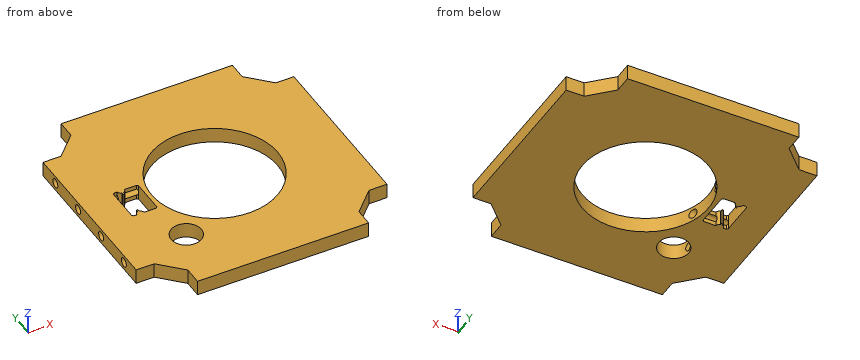
Autodesk Inventor part; units mm, degrees
ref_plane "Work Plane1" through (0, 0, 10) normal (0, 0, 1) x (1, 0, 0)
ref_plane "YZ Plane" through (0, 0, 0) normal (1, 0, 0) x (0, 1, 0)
ref_plane "XZ Plane" through (0, 0, 0) normal (0, 1, 0) x (-1, 0, 0)
ref_plane "Work Plane1" through (0, 0, 10) normal (0, 0, 1) x (1, 0, 0)
sketch "Sketch1" plane through (0, 0, 10) normal (0, 0, 1) x (1, 0, 0)
  line L0 (-4.0299, -0.3538) -> (-2.2322, 1.4439) construction
  arc A0 (-1.4439, 2.2322) -> (-2.2322, 1.4439) centre (-0.9299, 0.9299) ccw construction
  line L1 (-1.4439, 2.2322) -> (0.3538, 4.0299) construction
  line L2 (-37.8299, 42.8299) -> (-37.8299, 37.8299) construction
  line L3 (-37.8299, 37.8299) -> (-42.9208, 37.8299) construction
  line L4 (-37.8299, 42.2137) -> (-37.8299, 45.8299) construction
  line L5 (-37.8299, 45.8299) -> (-4.0299, 45.8299) construction
  line L6 (-4.0299, 45.8299) -> (-4.0299, 42.2137) construction
  line L7 (-4.0299, 4.0299) -> (0.3538, 4.0299)
  circle A1 centre (-20.9299, 20.9299) radius 17.5
  line L8 (-20.9299, 58.9723) -> (17.1124, 20.9299) construction
  line L9 (17.1124, 20.9299) -> (-20.9299, -17.1124) construction
  line L10 (-20.9299, -17.1124) -> (-58.9723, 20.9299) construction
  line L11 (-58.9723, 20.9299) -> (-20.9299, 58.9723) construction
  line L12 (-20.9299, 58.9723) -> (-20.9299, -17.1124) construction
  line L13 (17.1124, 20.9299) -> (-58.9723, 20.9299) construction
  line L14 (-20.9299, 58.9723) -> (32.8701, 58.9723) construction
  line L15 (-43.4299, 43.4299) -> (1.5701, 43.4299) construction
  line L16 (1.5701, 43.4299) -> (1.5701, -1.5701) construction
  line L17 (1.5701, -1.5701) -> (-43.4299, -1.5701) construction
  line L18 (-43.4299, -1.5701) -> (-43.4299, 43.4299) construction
  line L19 (-43.4299, 43.4299) -> (1.5701, -1.5701) construction
  line L20 (1.5701, 43.4299) -> (-43.4299, -1.5701) construction
  line L21 (-43.4299, 5.3876) -> (-43.4299, 36.4723)
  line L22 (-43.4299, 36.4723) -> (-36.4723, 43.4299)
  line L23 (-36.4723, 43.4299) -> (-5.3876, 43.4299)
  line L24 (-5.3876, 43.4299) -> (1.5701, 36.4723)
  line L25 (1.5701, 36.4723) -> (1.5701, 5.3876)
  line L26 (1.5701, 5.3876) -> (-5.3876, -1.5701)
  line L27 (-5.3876, -1.5701) -> (-36.4723, -1.5701)
  line L28 (-36.4723, -1.5701) -> (-43.4299, 5.3876)
  line L29 (-4.0299, 42.2137) -> (-37.8299, 42.2137)
  line L30 (-4.0299, -0.3538) -> (-4.0299, 4.0299)
  circle A2 centre (-20.9299, 20.9299) radius 1.5
  line L31 (-10.9299, 10.9299) -> (-30.9299, 10.9299) construction
  line L32 (-30.9299, 10.9299) -> (-30.9299, 30.9299) construction
  line L33 (-30.9299, 30.9299) -> (-10.9299, 30.9299) construction
  line L34 (-10.9299, 30.9299) -> (-10.9299, 10.9299) construction
  line L35 (-10.9299, 10.9299) -> (-30.9299, 30.9299) construction
  line L36 (-30.9299, 10.9299) -> (-10.9299, 30.9299) construction
  circle A3 centre (-30.9299, 30.9299) radius 1.4
  circle A4 centre (-30.9299, 10.9299) radius 1.4
  circle A5 centre (-10.9299, 10.9299) radius 1.4
  line L37 (-45.8299, 37.8299) -> (-42.0723, 37.8299) construction
  line L38 (-42.1723, 37.7299) -> (-45.8299, 37.7299)
  line L39 (-45.8299, 37.7299) -> (-45.8299, 4.1299)
  line L40 (-45.8299, 4.1299) -> (-42.1723, 4.1299)
  line L41 (-42.1723, 4.1299) -> (-42.1723, 37.7299)
  line L42 (-45.8299, 4.0299) -> (-42.0723, 4.0299) construction
  line L43 (-45.8299, 37.8299) -> (-42.0723, 37.8299)
  line L44 (-37.7299, 45.8299) -> (-4.1299, 45.8299)
  line L45 (-4.1299, 45.8299) -> (-4.1299, 42.1723)
  line L46 (-4.1299, 42.1723) -> (-37.7299, 42.1723)
  line L47 (-37.7299, 42.1723) -> (-37.7299, 45.8299)
  line L48 (0.4701, 37.8299) -> (0.4701, 4.0299) construction
  line L49 (0.4701, 4.0299) -> (3.9701, 4.0299) construction
  line L50 (3.9701, 37.8299) -> (3.9701, 4.0299) construction
  line L51 (0.4701, 37.8299) -> (3.9701, 37.8299) construction
  line L52 (-45.8299, -3.9701) -> (-4.0299, -3.9701) construction
  line L53 (0.3124, 37.7299) -> (3.9701, 37.7299)
  line L54 (3.9701, 37.7299) -> (3.9701, 4.1299)
  line L55 (3.9701, 4.1299) -> (0.3124, 4.1299)
  line L56 (0.3124, 4.1299) -> (0.3124, 37.7299)
  line L57 (-4.1713, -0.3538) -> (-37.7299, -0.3538)
  line L58 (-37.7299, -0.3538) -> (-37.7299, -3.9701)
  line L59 (-37.7299, -3.9701) -> (-4.1713, -3.9701)
  line L60 (-4.1713, -3.9701) -> (-4.1713, -0.3538)
  point P0 (-37.8299, 4.0299)
  dimension "d18" = 53.8
  dimension "d19" = 45
  dimension "d20" = 53.8
  dimension "d21" = 45
  dimension "d22" = 45
  dimension "d30" = 20
  dimension "d31" = 20
  dimension "d32" = 2.8
  dimension "d33" = 2.8
  dimension "d34" = 2.8
  dimension "d35" = 3
  dimension "d36" = 0.1
  dimension "d37" = 0.1
  dimension "d38" = 0.1
  dimension "d39" = 0.1
extrude "Extrusion1" add sketch "Sketch1" along normal blind 3 contours L30 L26 L57 L28 L41 L22 L46 L24 L56 L7 | L7 L26 L30 | L56 L24 L25 L26 | L26 L25 L24 L53 L54 L55 | L60 L59 L58 L57 L28 L27 L26 | L26 L27 L28 L57 | L46 L22 L29 L24 | L24 L29 L45 | L40 L39 L38 L22 L21 L28 | L28 L21 L22 L41 | L29 L22 L23 L24 | L24 L23 L22 L29 L47 L44 L45 | L47 L29 L22 | A1 | A2 | A3 | A4 | A5
sketch "Skizze4" plane through (0, 0, 13) normal (0, 0, 1) x (1, 0, 0)
  line L0 (-37.7299, 42.1723) -> (-42.1723, 37.7299)
  line L1 (-42.1723, 37.7299) -> (-45.8299, 37.7299)
  line L2 (-45.8299, 37.7299) -> (-45.8299, 4.1299) construction
  line L3 (-45.8299, 4.1299) -> (-42.1723, 4.1299)
  line L4 (-42.1723, 4.1299) -> (-37.6885, -0.3538)
  line L5 (-37.6885, -0.3538) -> (-37.7299, -0.3538)
  line L6 (-37.7299, -0.3538) -> (-37.7299, -3.9701)
  line L7 (-37.7299, -3.9701) -> (-4.1713, -3.9701) construction
  line L8 (-4.1713, -3.9701) -> (-4.1713, -0.3538)
  line L9 (-4.1713, -0.3538) -> (0.3124, 4.1299)
  line L10 (0.3124, 4.1299) -> (3.9701, 4.1299)
  line L11 (3.9701, 4.1299) -> (3.9701, 37.7299) construction
  line L12 (3.9701, 37.7299) -> (0.3124, 37.7299)
  line L13 (0.3124, 37.7299) -> (-4.1299, 42.1723)
  line L14 (-4.1299, 42.1723) -> (-4.1299, 45.8299)
  line L15 (-4.1299, 45.8299) -> (-37.7299, 45.8299) construction
  line L16 (-37.7299, 45.8299) -> (-37.7299, 42.1723)
  line L17 (-37.9299, 46.0299) -> (-3.9299, 46.0299) construction
  line L18 (-3.9299, 46.0299) -> (-3.9299, 42.2551)
  line L19 (-3.9299, 42.2551) -> (0.3953, 37.9299)
  line L20 (0.3953, 37.9299) -> (4.1701, 37.9299)
  line L21 (4.1701, 37.9299) -> (4.1701, 3.9299) construction
  line L22 (4.1701, 3.9299) -> (0.3953, 3.9299)
  line L23 (0.3953, 3.9299) -> (-3.9713, -0.4367)
  line L24 (-3.9713, -0.4367) -> (-3.9713, -4.1701)
  line L25 (-3.9713, -4.1701) -> (-37.9299, -4.1701) construction
  line L26 (-37.9299, -4.1701) -> (-37.9299, -0.3953)
  line L27 (-37.9299, -0.3953) -> (-42.2551, 3.9299)
  line L28 (-42.2551, 3.9299) -> (-46.0299, 3.9299)
  line L29 (-46.0299, 3.9299) -> (-46.0299, 37.9299) construction
  line L30 (-46.0299, 37.9299) -> (-42.2551, 37.9299)
  line L31 (-42.2551, 37.9299) -> (-37.9299, 42.2551)
  line L32 (-37.9299, 42.2551) -> (-37.9299, 46.0299)
  line L33 (-45.8299, 37.7299) -> (-45.8299, 37.9299)
  line L34 (-4.1299, 45.8299) -> (-37.7299, 45.8299)
  line L35 (-37.7299, 45.8299) -> (-37.9299, 45.8299)
  line L36 (-4.1299, 45.8299) -> (-3.9299, 45.8299)
  line L37 (3.9701, 37.7299) -> (3.9701, 37.9299)
  line L38 (3.9701, 4.1299) -> (3.9701, 37.7299)
  line L39 (3.9701, 4.1299) -> (3.9701, 3.9299)
  line L40 (-4.1713, -3.9701) -> (-3.9713, -3.9701)
  line L41 (-37.7299, -3.9701) -> (-37.9299, -3.9701)
  line L42 (-45.8299, 4.1299) -> (-45.8299, 3.9299)
  point P0 (0, 0)
  dimension "d40" = 0.2
extrude "IM_offset" add sketch "Skizze4" against normal up to surface (3 mm away)
ref_plane "Arbeitsebene5" through (-20.9299, 3.9299, 10) normal (1, 0, 0) x (0, 0, -1)
ref_plane "Arbeitsebene6" through (-37.9299, 20.9299, 10) normal (0, 1, 0) x (1, 0, 0)
sketch "Skizze25" plane through (0, 0, 13) normal (0, 0, 1) x (1, 0, 0)
  arc A0 (-37.9299, 18.0899) -> (-38.4737, 17.4299) centre (-37.6799, 17.3299) ccw
  line L0 (-37.9299, 18.0899) -> (-37.9299, 18.5899)
  line L1 (-37.9299, 18.5899) -> (-37.4299, 18.5899)
  line L2 (-37.4299, 18.5899) -> (-37.4299, 18.0899)
  arc A1 (-36.8862, 17.4299) -> (-37.4299, 18.0899) centre (-37.6799, 17.3299) ccw
  line L3 (-36.8862, 17.4299) -> (-34.5799, 17.4299)
  line L4 (-34.5799, 17.4299) -> (-34.3799, 17.6299)
  line L5 (-34.3799, 17.6299) -> (-34.3799, 24.2299)
  line L6 (-34.3799, 24.2299) -> (-34.5799, 24.4299)
  line L7 (-34.5799, 24.4299) -> (-36.8862, 24.4299)
  arc A2 (-37.4299, 23.77) -> (-36.8862, 24.4299) centre (-37.6799, 24.5299) ccw
  line L8 (-37.4299, 23.77) -> (-37.4299, 23.27)
  line L9 (-37.4299, 23.27) -> (-37.9299, 23.27)
  line L10 (-37.9299, 23.27) -> (-37.9299, 23.77)
  arc A3 (-38.4737, 24.4299) -> (-37.9299, 23.77) centre (-37.6799, 24.5299) ccw
  line L11 (-38.4737, 24.4299) -> (-38.9799, 24.4299)
  line L12 (-38.9799, 24.4299) -> (-39.1799, 24.2299)
  line L13 (-39.1799, 24.2299) -> (-39.1799, 17.6299)
  line L14 (-39.1799, 17.6299) -> (-38.9799, 17.4299)
  line L15 (-38.9799, 17.4299) -> (-38.4737, 17.4299)
  line L16 (-34.2799, 24.2713) -> (-34.2799, 17.5885)
  line L17 (-34.2799, 17.5885) -> (-34.5385, 17.3299)
  line L18 (-34.5385, 17.3299) -> (-36.9799, 17.3299)
  arc A4 (-36.9799, 17.3299) -> (-37.5299, 18.0137) centre (-37.6799, 17.3299) ccw
  line L19 (-37.5299, 18.0137) -> (-37.5299, 18.4899)
  line L20 (-37.5299, 18.4899) -> (-37.8299, 18.4899)
  line L21 (-37.8299, 18.4899) -> (-37.8299, 18.0137)
  arc A5 (-37.8299, 18.0137) -> (-38.3799, 17.3299) centre (-37.6799, 17.3299) ccw
  line L22 (-38.3799, 17.3299) -> (-39.0213, 17.3299)
  line L23 (-39.0213, 17.3299) -> (-39.2799, 17.5885)
  line L24 (-39.2799, 17.5885) -> (-39.2799, 24.2713)
  line L25 (-39.2799, 24.2713) -> (-39.0213, 24.5299)
  line L26 (-39.0213, 24.5299) -> (-38.3799, 24.5299)
  arc A6 (-38.3799, 24.5299) -> (-37.8299, 23.8462) centre (-37.6799, 24.5299) ccw
  line L27 (-37.8299, 23.8462) -> (-37.8299, 23.37)
  line L28 (-37.8299, 23.37) -> (-37.5299, 23.37)
  line L29 (-37.5299, 23.37) -> (-37.5299, 23.8462)
  arc A7 (-37.5299, 23.8462) -> (-36.9799, 24.5299) centre (-37.6799, 24.5299) ccw
  line L30 (-36.9799, 24.5299) -> (-34.5385, 24.5299)
  line L31 (-34.5385, 24.5299) -> (-34.2799, 24.2713)
  circle A8 centre (-21.0099, 20.9299) radius 10.125
  circle A9 centre (-21.0099, 20.9299) radius 12.5
  point P0 (0, 0)
  dimension "d150" = 0.1
  dimension "d151" = 25
extrude "Extrusion21" cut sketch "Skizze25" against normal blind 3 contours A0 L15 L14 L13 L12 L11 A3 L10 L9 L8 A2 L7 L6 L5 L4 L3 A1 L2 L1 L0 | L16 L17 L18 A4 L19 L20 L21 A5 L22 L23 L24 L25 L26 A6 L27 L28 L29 A7 L30 L31 | A8 | A9
sketch "Skizze26" plane through (-45.8299, 3.9299, 10) normal (-1, 0, 0) x (0, 0, 1)
  line L0 (0, 0) -> (0, 34)
  line L1 (3, 0) -> (0, 0)
  line L2 (3, 34) -> (3, 0)
  line L3 (3, 34) -> (0, 34)
  line L4 (3, 29.5) -> (0, 29.5)
  circle A0 centre (1.5, 29.5) radius 0.9
  line L5 (3, 4.5) -> (0, 4.5)
  circle A1 centre (1.5, 4.5) radius 0.9
  line L6 (36.97, 20.3) -> (-3.03, 20.3)
  line L7 (36.97, 13.7) -> (-3.03, 13.7)
  circle A2 centre (1.5, 21.2) radius 0.9
  circle A3 centre (1.5, 12.8) radius 0.9
  point P0 (-10, -3.9299)
  dimension "d154" = 1.8
  dimension "d155" = 1.8
  dimension "d158" = 1.8
  dimension "d159" = 1.8
extrude "Extrusion22" cut sketch "Skizze26" against normal blind 15 contours A3 | A1 L5 | L5 A1 | A2 | A0 L4 | L4 A0
sketch "Skizze27" plane through (0, 0, 10) normal (0, 0, -1) x (-1, 0, 0)
  arc A0 (36.9799, 24.5299) -> (37.5299, 23.8462) centre (37.6799, 24.5299) ccw
  line L0 (37.5299, 23.8462) -> (37.5299, 23.37)
  line L1 (37.5299, 23.37) -> (37.8299, 23.37)
  line L2 (37.8299, 23.37) -> (37.8299, 23.8462)
  arc A1 (37.8299, 23.8462) -> (38.3799, 24.5299) centre (37.6799, 24.5299) ccw
  line L3 (38.3799, 24.5299) -> (39.0213, 24.5299)
  line L4 (39.0213, 24.5299) -> (39.2799, 24.2713)
  line L5 (39.2799, 24.2713) -> (39.2799, 17.5885)
  line L6 (39.2799, 17.5885) -> (39.0213, 17.3299)
  line L7 (39.0213, 17.3299) -> (38.3799, 17.3299)
  arc A2 (38.3799, 17.3299) -> (37.8299, 18.0137) centre (37.6799, 17.3299) ccw
  line L8 (37.8299, 18.0137) -> (37.8299, 18.4899)
  line L9 (37.8299, 18.4899) -> (37.5299, 18.4899)
  line L10 (37.5299, 18.4899) -> (37.5299, 18.0137)
  arc A3 (37.5299, 18.0137) -> (36.9799, 17.3299) centre (37.6799, 17.3299) ccw
  line L11 (36.9799, 17.3299) -> (34.5385, 17.3299)
  line L12 (34.5385, 17.3299) -> (34.2799, 17.5885)
  line L13 (34.2799, 17.5885) -> (34.2799, 24.2713)
  line L14 (34.2799, 24.2713) -> (34.5385, 24.5299)
  line L15 (34.5385, 24.5299) -> (36.9799, 24.5299)
  circle A4 centre (21.0099, 20.9299) radius 12.5
  line L16 (3.9713, -3.9701) -> (37.9299, -3.9701)
  line L17 (37.9299, -3.9701) -> (37.9299, -0.3953)
  line L18 (37.9299, -0.3953) -> (42.2551, 3.9299)
  line L19 (42.2551, 3.9299) -> (45.8299, 3.9299)
  line L20 (45.8299, 3.9299) -> (45.8299, 37.9299)
  line L21 (45.8299, 37.9299) -> (42.2551, 37.9299)
  line L22 (42.2551, 37.9299) -> (37.9299, 42.2551)
  line L23 (37.9299, 42.2551) -> (37.9299, 45.8299)
  line L24 (37.9299, 45.8299) -> (3.9299, 45.8299)
  line L25 (3.9299, 45.8299) -> (3.9299, 42.2551)
  line L26 (3.9299, 42.2551) -> (-0.3953, 37.9299)
  line L27 (-0.3953, 37.9299) -> (-3.9701, 37.9299)
  line L28 (-3.9701, 37.9299) -> (-3.9701, 3.9299)
  line L29 (-3.9701, 3.9299) -> (-0.3953, 3.9299)
  line L30 (-0.3953, 3.9299) -> (3.9713, -0.4367)
  line L31 (3.9713, -0.4367) -> (3.9713, -3.9701)
  line L32 (37.9799, 3.9599) -> (37.9799, 43.7799)
  line L33 (37.9799, 3.9599) -> (3.8799, 3.9599)
  circle A5 centre (33.4322, 8.4277) radius 3
  circle A6 centre (33.4322, 8.4277) radius 1.4
  point P0 (0, 0)
  point P1 (35.8514, 12.3014)
  dimension "d160" = 6
extrude "Extrusion23" cut sketch "Skizze27" against normal blind 15 contours A5 | A6
properties part number "20_Cube_Insert_lineartranlator_mgn7_base_v3"
CAD build for the part. Positions are in the model's coordinates, mm. Give positions to 0.01 mm unless a question says otherwise; leave off trailing zeros. Order: outer loops, then holes, each group sorted by start corner. A loop starts at its lowest first (then second) coordinate and runs counter-clockwise, first axis right, second up.
(1) Saw through at B-B, the plane y = 30. Give the cut face in (x, z).
(2) Saw through at C-C, the plane y = 19.5. Give the cut face in (x, z).
(3) Saw through at A-A, the plane x = -14. Give the cut face in (y, z), then the cut area to 3 significant figures.
(4) Flat gauge pins, fed straight in: pin 1 (0.9 mm diameter, centred on y = 44, z = 11.5, fed in from +X); pin 2 (0.5 mm diameter, centred on y = 33.5, z = 12, fed in from -X); pin 3 (0.9 mm diameter, centred on y = -1.5, z = 11.5, fed in from -X); pin 4 (5 mm diameter, centred on x = -14, y = 17, fed in from +Z). Where does each tip first touch, or does it go through?
(5) Saw through at D-D, the plane y = 1. Give the cut face in (x, z), then the cut area to 3 significant figures.
(6) Drill centre lines: L1, parallel to Y at x = -37.75, z = 11.5; L2, parallel to Y at x = -35, z = 12.1; L3, parallel to Y at x = -31, z = 11.3. Where is each one in solid material? Low to high.
Results found:
1. outline: (-45.83, 10) - (-29.61, 10) - (-29.61, 13) - (-45.83, 13) - close; (-12.41, 10) - (3.97, 10) - (3.97, 13) - (-12.41, 13) - close
2. outline: (-45.83, 10) - (-39.28, 10) - (-39.28, 13) - (-45.83, 13) - close; (-34.28, 10) - (-33.43, 10) - (-33.43, 13) - (-34.28, 13) - close; (-8.59, 10) - (3.97, 10) - (3.97, 13) - (-8.59, 13) - close
3. outline: (-3.97, 10) - (10.58, 10) - (10.58, 13) - (-3.97, 13) - close; (31.28, 10) - (45.83, 10) - (45.83, 13) - (31.28, 13) - close
3. area: 87.3 mm2
4. pin 1: stops at x = -3.93
4. pin 2: stops at x = -30.83
4. pin 3: stops at x = -37.93
4. pin 4: passes through
5. outline: (-39.33, 10) - (-2.53, 10) - (-2.53, 13) - (-39.33, 13) - close
5. area: 110 mm2
6. L1: y = -3.97 to 7.53, 9.33 to 15.83, 17.63 to 18.49, 23.37 to 24.23, 26.03 to 32.53, 34.33 to 45.83
6. L2: y = -3.97 to 5.87, 10.99 to 16.06, 25.8 to 32.76, 34.1 to 45.83
6. L3: y = -3.97 to 6.67, 10.18 to 13.42, 28.44 to 32.55, 34.31 to 45.83
